Autodesk Fusion 360 part; units mm, degrees
sketch "Sketch1" plane through (0, 0, 0) normal (0, 1, 0) x (1, 0, 0)
  arc A0 (111.125, 0) -> (114.3, 3.175) centre (111.125, 3.175) ccw
  line L0 (0, 0) -> (114.3, 0)
  line L1 (114.3, 0) -> (114.3, 101.6)
  arc A1 (3.175, 101.6) -> (0, 98.425) centre (3.175, 98.425) ccw
  arc A2 (0, 3.175) -> (3.175, 0) centre (3.175, 3.175) ccw
  circle A3 centre (25.4, 50.8) radius 3.175
  circle A4 centre (88.9, 50.8) radius 3.175
  line L2 (0, 101.6) -> (0, 0)
  line L3 (114.3, 101.6) -> (0, 101.6)
  arc A5 (114.3, 98.425) -> (111.125, 101.6) centre (111.125, 98.425) ccw
  line L4 (8.1496, 70.993) -> (8.1496, 30.988)
  line L5 (106.1504, 70.993) -> (8.1496, 70.993)
  line L6 (8.1496, 30.988) -> (106.1504, 30.988)
  line L7 (106.1504, 80.6374) -> (8.1496, 80.6374)
  line L8 (8.1496, 20.6375) -> (106.1504, 20.6375)
  line L9 (106.1504, 20.6375) -> (106.1504, 80.6374)
  line L10 (8.1496, 80.6374) -> (8.1496, 20.6375)
  line L11 (106.1504, 30.988) -> (106.1504, 70.993)
  circle A6 centre (65.3796, 13.716) radius 3.683
  circle A7 centre (48.4378, 13.716) radius 3.683
  circle A8 centre (82.3214, 13.716) radius 3.683
  circle A9 centre (31.4198, 13.716) radius 3.683
  circle A10 centre (103.6498, 23.241) radius 1.778
  circle A11 centre (10.6528, 23.241) radius 1.778
  circle A12 centre (10.6528, 78.2422) radius 1.778
  circle A13 centre (103.6498, 78.2422) radius 1.778
  circle A14 centre (9.525, 92.075) radius 1.778
  circle A15 centre (9.525, 9.525) radius 1.778
  circle A16 centre (104.775, 9.525) radius 1.778
  circle A17 centre (106.045, 92.075) radius 1.778
extrude "Extrude1" add sketch "Sketch1" along normal blind 2.9972 contours A0 L0 L1 A1 A2 L2 L3 A5 | L5 L7 L9 L10 | L6 L8 L9 L10
The model under review builds one solid part; all positions refer to its coordinate system, in mm. A direction names the side the tool comes from. Give positions to 0.01 mm unless a question says otherwise; leave off trailing zeros. Write each loop counter-clockwise with the first axis right and the second up, starting at its lowest first coordinate (ties: lowest second). Pieces come first, ordered by that corner, then holes.
(1) Consider section B-B, the plane x = 93. Give the boundary of the cut face in (y, z), and give its area (3 significant figures).
(2) To check wall thickness, follow L1, parallel to Z at x = 95, y = 2.3; L2, parallel to Z at x = 80.5, y = 1.2; L3, parallel to X at y = 2.45, z = -23.5. State the ranges of each line that lie inside material, in increasing order.
(3) Consider section A-A, the plane z = -56.5. Give the boundary of the cut face in (x, y), and give its area (3 significant figures).
(4) Tool access review of faces 1 (the cylindrical face through (113.35, 1.48, -100.69)), 2 (the flat face through (8.15, 1, -51)): name each direction out of +Z, -Z, +X, -X, +Y, -Y from which nothing blocks a thin tool from reaching the whole face with its end or side.
(5) The part is to be moulded in two halves that separate along Z. For faces 3 (the flat face through (56, 1, -30.988)), 4 (the flat face through (58, 1, -101.6)), 5 (the cylindrical face through (0.95, 1.48, -0.91)), say which applies: released by +Z, released by -Z, zero draft, split by the parting line, or undercut.
(6) Consider section D-D, the plane z = -15.5. Give the boundary of the cut face in (x, y), and give its area (3 significant figures).
(7) Consider section C-C, the plane y = 1.9. Give the number of separate pieces and of enclosed holes in the cut face, and give its area (3 significant figures).
Returned:
1. outline: (0, -101.6) - (3, -101.6) - (3, -70.99) - (0, -70.99) - close; (0, -30.99) - (3, -30.99) - (3, 0) - (0, 0) - close
1. area: 185 mm2
2. L1: z = -101.6 to -70.99, -30.99 to 0
2. L2: z = -101.6 to -70.99, -30.99 to -16.92, -10.51 to 0
2. L3: x = 0 to 8.89, 12.41 to 101.89, 105.41 to 114.3
3. outline: (0, 0) - (8.15, 0) - (8.15, 3) - (0, 3) - close; (106.15, 0) - (114.3, 0) - (114.3, 3) - (106.15, 3) - close
3. area: 48.9 mm2
4. face 1: -Z, +X, +Y, -Y
4. face 2: +Y, -Y
5. face 3: undercut
5. face 4: released by -Z
5. face 5: released by +Z
6. outline: (0, 0) - (28.2, 0) - (28.2, 3) - (0, 3) - close; (34.64, 0) - (45.22, 0) - (45.22, 3) - (34.64, 3) - close; (51.66, 0) - (62.16, 0) - (62.16, 3) - (51.66, 3) - close; (68.6, 0) - (79.1, 0) - (79.1, 3) - (68.6, 3) - close; (85.54, 0) - (114.3, 0) - (114.3, 3) - (85.54, 3) - close
6. area: 265 mm2
7. separate pieces: 1
7. enclosed holes: 13
7. area: 7,430 mm2
